```python
from build123d import *

# Parameters (mm, degrees)
F0_W     = 280
F0_H     = 420
F1_DEPTH = 18
F2_W     = 280
F2_H     = 18
F2_H_2   = 7
F3_DEPTH = 5


with BuildPart() as f1:
    # F0 (on Right) → F1 (new body)
    with BuildSketch(Plane.YZ):
        with Locations((140, 210)):
            Rectangle(F0_W, F0_H)
    extrude(amount=F1_DEPTH)

    # F2 (on face) → F3 (cut)
    with BuildSketch(Plane(origin=(0, 0, 0), x_dir=(0, -1, 0), z_dir=(-1, 0, 0))):
        with Locations((-140, 79)):
            Rectangle(F2_W, F2_H)
        with Locations((-140, 161.5)):
            Rectangle(F2_W, F2_H_2)
        with Locations((-140, 238.5)):
            Rectangle(F2_W, F2_H_2)
        with Locations((-140, 315.5)):
            Rectangle(F2_W, F2_H_2)
        with Locations((-140, 398)):
            Rectangle(F2_W, F2_H)
    extrude(amount=-F3_DEPTH, mode=Mode.SUBTRACT)


solid = f1.part
```
Geometry check sheet. Reference: the model listing, model coordinates, mm. Give positions to 0.01 mm unless a question says otherwise; leave off trailing zeros. Loops run counter-clockwise (first coordinate to the right, second up) from the corner with the lowest first, then second, coordinate; pieces in that order, holes last. Notation, with made-up numbers: (19, 81.5) - (23, 81.5) arc R27 cw to (23, 105.5) - close; hole circle Ø5 at (-33, 37.25). An arc over 180 degrees is marked (long way). Use CSV: the item, a comma, the result in double quotes. Start each with the question number.
Q1. Release check for a two-part mould opening along Z. For faces 1 (the face through (5, 142, 398)), 2 (the face through (0, 138, 200)), 3 (the face through (5, 142, 79)), 4 (the face through (9, 138, 420)) record: +Z half, -Z half, draft (parallel to the pull), parting line (faces both ways), or undercut.
Q2. Scan line: probe 1 along Z at (x, y) = (1, 146.5). Record every from-to range of solid material in increasing order. Write a range as from..to.
Q3. Section check A-A, the plane y = 239. Record the cut outline in (x, z), and give its area (4 significant figures).
Q4. Go/stop test with flat-tipped pins: pin 1 Ø3.5 at (y, z) = (162, 162) entering from -X; pin 2 Ø7.5 at (y, z) = (192, 317) entering from -X. Record where each tip stops, or that it passes through.
Findings below:
1,face 1,"undercut"
1,face 2,"draft"
1,face 3,"undercut"
1,face 4,"+Z half"
2,probe 1,"z = 0..70, 88..158, 165..235, 242..312, 319..389, 407..420"
3,outline,"(0, 0) - (18, 0) - (18, 420) - (0, 420) - (0, 407) - (5, 407) - (5, 389) - (0, 389) - (0, 319) - (5, 319) - (5, 312) - (0, 312) - (0, 242) - (5, 242) - (5, 235) - (0, 235) - (0, 165) - (5, 165) - (5, 158) - (0, 158) - (0, 88) - (5, 88) - (5, 70) - (0, 70) - close"
3,area,"7,275 mm^2"
4,pin 1,"stops at x = 5"
4,pin 2,"stops at x = 0"
